```python
from build123d import *

# Parameters (mm, degrees)
BOSS_EXTRU_1_DEPTH      = 40
ESQUISSE2_R             = 8
ENL_V_MAT_EXTRU_1_DEPTH = 190.883457354
ESQUISSE3_R             = 8
ENL_V_MAT_EXTRU_2_DEPTH = 181.562836456
BOSS_EXTRU_2_DEPTH      = 6.35
BOSS_EXTRU_3_START      = 6.35
BOSS_EXTRU_3_DEPTH      = 6.35
ENL_V_START             = -9.5
ENL_V_MAT_EXTRU_3_DEPTH = 9.5
ENL_V_MAT_EXTRU_6_DEPTH = 9.5


with BuildPart() as part:
    # Esquisse1 → Boss.-Extru.1 (new body)
    with BuildSketch(Plane.XY):
        with BuildLine():
            ThreePointArc((-10.389343798, 19.957743747), (6.765880489, 21.458631392), (19.957743747, 10.389343798))
            Line((19.957743747, 10.389343798), (-16.981934979, 81.349806406))
            Line((-16.981934979, 81.349806406), (-28.734828519, 75.231637281))
            Line((-28.734828519, 75.231637281), (-49.975475061, 116.034539653))
            Line((-49.975475061, 116.034539653), (-58.180325268, 111.76336498))
            Line((-58.180325268, 111.76336498), (-10.389343798, 19.957743747))
        make_face()
        with BuildLine():
            ThreePointArc((-22.5, 0), (-19.23551709, 11.672398309), (-10.389343798, 19.957743747))
            Line((-10.389343798, 19.957743747), (-58.180325268, 111.76336498))
            Line((-58.180325268, 111.76336498), (-66.385175475, 107.492190308))
            Line((-66.385175475, 107.492190308), (-45.144528933, 66.689287936))
            Line((-45.144528933, 66.689287936), (-88.25, 44.25))
            Line((-88.25, 44.25), (-88.25, 9.25))
            Line((-88.25, 9.25), (-140, 9.25))
            Line((-140, 9.25), (-140, 0))
            Line((-140, 0), (-22.5, 0))
        make_face()
        with BuildLine():
            Line((-88.25, -22.560492565), (0.015421683, -22.499994715))
            ThreePointArc((0.015421683, -22.499994715), (-15.904449254, -15.915354031), (-22.5, 0))
            Line((-22.5, 0), (-140, 0))
            Line((-140, 0), (-140, -9.25))
            Line((-140, -9.25), (-88.25, -9.25))
            Line((-88.25, -9.25), (-88.25, -22.560492565))
        make_face()
        with BuildLine():
            ThreePointArc((22.5, 0), (21.855196571, 5.347932577), (19.957743747, 10.389343798))
            ThreePointArc((19.957743747, 10.389343798), (6.765880489, 21.458631392), (-10.389343798, 19.957743747))
            Line((-10.389343798, 19.957743747), (-4.386611826, 8.426602915))
            ThreePointArc((-4.386611826, 8.426602915), (4.928345953, 8.121662771), (9.5, 0))
            ThreePointArc((9.5, 0), (0, -9.5), (-9.5, 0))
            Line((-9.5, 0), (-22.5, 0))
            ThreePointArc((-22.5, 0), (-15.904449254, -15.915354031), (0.015421683, -22.499994715))
            ThreePointArc((0.015421683, -22.499994715), (15.915354031, -15.904449254), (22.5, 0))
        make_face()
        with BuildLine():
            Line((-4.386611826, 8.426602915), (-10.389343798, 19.957743747))
            ThreePointArc((-10.389343798, 19.957743747), (-19.23551709, 11.672398309), (-22.5, 0))
            Line((-22.5, 0), (-9.5, 0))
            ThreePointArc((-9.5, 0), (-8.121662771, 4.928345953), (-4.386611826, 8.426602915))
        make_face()
        with BuildLine():
            ThreePointArc((22.5, 0), (21.855196571, 5.347932577), (19.957743747, 10.389343798))
            ThreePointArc((19.957743747, 10.389343798), (6.765880489, 21.458631392), (-10.389343798, 19.957743747))
            Line((-10.389343798, 19.957743747), (-4.386611826, 8.426602915))
            ThreePointArc((-4.386611826, 8.426602915), (4.928345953, 8.121662771), (9.5, 0))
            ThreePointArc((9.5, 0), (0, -9.5), (-9.5, 0))
            Line((-9.5, 0), (-22.5, 0))
            ThreePointArc((-22.5, 0), (-15.904449254, -15.915354031), (0.015421683, -22.499994715))
            ThreePointArc((0.015421683, -22.499994715), (15.915354031, -15.904449254), (22.5, 0))
        make_face()
        with BuildLine():
            Line((-4.386611826, 8.426602915), (-10.389343798, 19.957743747))
            ThreePointArc((-10.389343798, 19.957743747), (-19.23551709, 11.672398309), (-22.5, 0))
            Line((-22.5, 0), (-9.5, 0))
            ThreePointArc((-9.5, 0), (-8.121662771, 4.928345953), (-4.386611826, 8.426602915))
        make_face()
    extrude(amount=BOSS_EXTRU_1_DEPTH)

    # Esquisse2 → Enlèv. mat.-Extru.1 (cut, through all)
    with BuildSketch(Plane(origin=(8.204850207, 4.271174672, 0), x_dir=(0, 0, -1), z_dir=(0.8870108331782228, 0.4617486132350319, 0))):
        with Locations(Location((-20, 106, 0), (0, 0, 90))):
            Circle(ESQUISSE2_R)
        with BuildLine():
            ThreePointArc((-40, 106), (-34.142135624, 120.142135624), (-20, 126))
            Line((-20, 126), (-40, 126))
            Line((-40, 126), (-40, 106))
        make_face()
        with BuildLine():
            ThreePointArc((-20, 126), (-5.857864376, 120.142135624), (0, 106))
            Line((0, 106), (0, 126))
            Line((0, 126), (-20, 126))
        make_face()
    extrude(amount=-ENL_V_MAT_EXTRU_1_DEPTH, mode=Mode.SUBTRACT)

    # Esquisse3 → Enlèv. mat.-Extru.2 (cut, through all)
    with BuildSketch(Plane(origin=(0, 9.25, 0), x_dir=(1, 0, 0), z_dir=(0, 1, 0))):
        with BuildLine():
            ThreePointArc((-140, -20), (-134.142135624, -5.857864376), (-120, 0))
            Line((-120, 0), (-140, 0))
            Line((-140, 0), (-140, -20))
        make_face()
        with BuildLine():
            ThreePointArc((-120, -40), (-134.142135624, -34.142135624), (-140, -20))
            Line((-140, -20), (-140, -40))
            Line((-140, -40), (-120, -40))
        make_face()
        with Locations(Location((-120, -20, 0), (0, 0, 180))):
            Circle(ESQUISSE3_R)
    extrude(amount=-ENL_V_MAT_EXTRU_2_DEPTH, mode=Mode.SUBTRACT)

    # Esquisse4 → Boss.-Extru.2 (add)
    with BuildSketch(Plane.XY.offset(40)):
        with BuildLine():
            ThreePointArc((22.5, 0), (21.855196571, 5.347932577), (19.957743747, 10.389343798))
            ThreePointArc((19.957743747, 10.389343798), (6.765880489, 21.458631392), (-10.389343798, 19.957743747))
            Line((-10.389343798, 19.957743747), (-4.386611826, 8.426602915))
            ThreePointArc((-4.386611826, 8.426602915), (4.928345953, 8.121662771), (9.5, 0))
            ThreePointArc((9.5, 0), (0, -9.5), (-9.5, 0))
            Line((-9.5, 0), (-22.5, 0))
            ThreePointArc((-22.5, 0), (-15.904449254, -15.915354031), (0.015421683, -22.499994715))
            ThreePointArc((0.015421683, -22.499994715), (15.915354031, -15.904449254), (22.5, 0))
        make_face()
        with BuildLine():
            ThreePointArc((22.5, 0), (21.855196571, 5.347932577), (19.957743747, 10.389343798))
            ThreePointArc((19.957743747, 10.389343798), (6.765880489, 21.458631392), (-10.389343798, 19.957743747))
            Line((-10.389343798, 19.957743747), (-4.386611826, 8.426602915))
            ThreePointArc((-4.386611826, 8.426602915), (4.928345953, 8.121662771), (9.5, 0))
            ThreePointArc((9.5, 0), (0, -9.5), (-9.5, 0))
            Line((-9.5, 0), (-22.5, 0))
            ThreePointArc((-22.5, 0), (-15.904449254, -15.915354031), (0.015421683, -22.499994715))
            ThreePointArc((0.015421683, -22.499994715), (15.915354031, -15.904449254), (22.5, 0))
        make_face()
        with BuildLine():
            Line((-4.386611826, 8.426602915), (-10.389343798, 19.957743747))
            ThreePointArc((-10.389343798, 19.957743747), (-19.23551709, 11.672398309), (-22.5, 0))
            Line((-22.5, 0), (-9.5, 0))
            ThreePointArc((-9.5, 0), (-8.121662771, 4.928345953), (-4.386611826, 8.426602915))
        make_face()
    extrude(amount=BOSS_EXTRU_2_DEPTH)

    # Esquisse5 → Boss.-Extru.3 (add)
    with BuildSketch(Plane(origin=(0, 0, 0), x_dir=(-1, 0, 0), z_dir=(0, 0, -1)).offset(BOSS_EXTRU_3_START)):
        with BuildLine():
            ThreePointArc((10.389343798, 19.957743747), (-6.765880489, 21.458631392), (-19.957743747, 10.389343798))
            ThreePointArc((-19.957743747, 10.389343798), (-19.239516139, -11.665805533), (-0.015421683, -22.499994715))
            ThreePointArc((-0.015421683, -22.499994715), (15.904449254, -15.915354031), (22.5, 0))
            Line((22.5, 0), (9.5, 0))
            ThreePointArc((9.5, 0), (-8.121662771, -4.928345953), (4.386611826, 8.426602915))
            Line((4.386611826, 8.426602915), (10.389343798, 19.957743747))
        make_face()
        with BuildLine():
            ThreePointArc((22.5, 0), (19.23551709, 11.672398309), (10.389343798, 19.957743747))
            Line((10.389343798, 19.957743747), (4.386611826, 8.426602915))
            ThreePointArc((4.386611826, 8.426602915), (8.121662771, 4.928345953), (9.5, 0))
            Line((9.5, 0), (22.5, 0))
        make_face()
        with BuildLine():
            ThreePointArc((10.389343798, 19.957743747), (-6.765880489, 21.458631392), (-19.957743747, 10.389343798))
            ThreePointArc((-19.957743747, 10.389343798), (-19.239516139, -11.665805533), (-0.015421683, -22.499994715))
            ThreePointArc((-0.015421683, -22.499994715), (15.904449254, -15.915354031), (22.5, 0))
            Line((22.5, 0), (9.5, 0))
            ThreePointArc((9.5, 0), (-8.121662771, -4.928345953), (4.386611826, 8.426602915))
            Line((4.386611826, 8.426602915), (10.389343798, 19.957743747))
        make_face()
    extrude(amount=-BOSS_EXTRU_3_DEPTH)

    # Esquisse6 → Enlèv. mat.-Extru.3 (cut)
    with BuildSketch(Plane.XY.offset(40).offset(ENL_V_START)):
        with BuildLine():
            Line((19.957743747, 10.389343798), (-12.595323154, 72.923203491))
            Line((-12.595323154, 72.923203491), (-17.695635444, 70.268148965))
            ThreePointArc((-17.695635444, 70.268148965), (-21.385397976, 65.870861212), (-20.885102094, 60.152453117))
            Line((-20.885102094, 60.152453117), (-3.287380782, 26.347545001))
            ThreePointArc((-3.287380782, 26.347545001), (-0.879642567, 23.627512536), (2.52390035, 22.3579947))
            ThreePointArc((2.52390035, 22.3579947), (12.734529101, 18.549441193), (19.957743747, 10.389343798))
        make_face()
        with BuildLine():
            Line((-78.75, -22.553981187), (0.015421683, -22.499994715))
            ThreePointArc((0.015421683, -22.499994715), (-10.566597122, -19.864466398), (-18.666376021, -12.5625))
            ThreePointArc((-18.666376021, -12.5625), (-21.364033316, -10.129718662), (-24.888501361, -9.25))
            Line((-24.888501361, -9.25), (-71.25, -9.25))
            ThreePointArc((-71.25, -9.25), (-76.553300859, -11.446699141), (-78.75, -16.75))
            Line((-78.75, -16.75), (-78.75, -22.553981187))
        make_face()
        with BuildLine():
            Line((-20.950564458, 20.213114599), (-37.294802508, 51.610103772))
            ThreePointArc((-37.294802508, 51.610103772), (-41.69209026, 55.299866303), (-47.410498356, 54.799570422))
            Line((-47.410498356, 54.799570422), (-74.713114599, 40.586728011))
            ThreePointArc((-74.713114599, 40.586728011), (-77.66183903, 37.824946199), (-78.75, 33.934146763))
            Line((-78.75, 33.934146763), (-78.75, 16.75))
            ThreePointArc((-78.75, 16.75), (-76.553300859, 11.446699141), (-71.25, 9.25))
            Line((-71.25, 9.25), (-27.603145707, 9.25))
            ThreePointArc((-27.603145707, 9.25), (-21.191306677, 12.859200564), (-20.950564458, 20.213114599))
        make_face()
    extrude(amount=ENL_V_MAT_EXTRU_3_DEPTH, mode=Mode.SUBTRACT)

    # Esquisse9 → Enlèv. mat.-Extru.6 (cut)
    with BuildSketch(Plane(origin=(0, 0, 0), x_dir=(-1, 0, 0), z_dir=(0, 0, -1))):
        with BuildLine():
            ThreePointArc((-19.957743747, 10.389343798), (-12.734529101, 18.549441193), (-2.52390035, 22.3579947))
            ThreePointArc((-2.52390035, 22.3579947), (0.879642567, 23.627512536), (3.287380782, 26.347545001))
            Line((3.287380782, 26.347545001), (20.885102094, 60.152453117))
            ThreePointArc((20.885102094, 60.152453117), (21.385397976, 65.870861212), (17.695635444, 70.268148965))
            Line((17.695635444, 70.268148965), (12.595323154, 72.923203491))
            Line((12.595323154, 72.923203491), (-19.957743747, 10.389343798))
        make_face()
        with BuildLine():
            Line((47.410498356, 54.799570422), (74.713114599, 40.586728011))
            ThreePointArc((74.713114599, 40.586728011), (77.66183903, 37.824946199), (78.75, 33.934146763))
            Line((78.75, 33.934146763), (78.75, 16.75))
            ThreePointArc((78.75, 16.75), (76.553300859, 11.446699141), (71.25, 9.25))
            Line((71.25, 9.25), (27.603145707, 9.25))
            ThreePointArc((27.603145707, 9.25), (21.191306677, 12.859200564), (20.950564458, 20.213114599))
            Line((20.950564458, 20.213114599), (37.294802508, 51.610103772))
            ThreePointArc((37.294802508, 51.610103772), (41.69209026, 55.299866303), (47.410498356, 54.799570422))
        make_face()
        with BuildLine():
            Line((71.25, -9.25), (24.888501361, -9.25))
            ThreePointArc((24.888501361, -9.25), (21.364033316, -10.129718662), (18.666376021, -12.5625))
            ThreePointArc((18.666376021, -12.5625), (10.566597122, -19.864466398), (-0.015421683, -22.499994715))
            Line((-0.015421683, -22.499994715), (78.75, -22.553981187))
            Line((78.75, -22.553981187), (78.75, -16.75))
            ThreePointArc((78.75, -16.75), (76.553300859, -11.446699141), (71.25, -9.25))
        make_face()
    extrude(amount=-ENL_V_MAT_EXTRU_6_DEPTH, mode=Mode.SUBTRACT)


solid = part.part
```
Part model, mm, in its own coordinate system. A direction names the side the tool comes from. Give positions to 0.01 mm unless a question says otherwise; leave off trailing zeros. Order: outer loops, then holes, each group sorted by start corner. A loop starts at its lowest first (then second) coordinate and runs counter-clockwise, first axis right, second up. Notation, with made-up numbers: M 44.25,35.5 L 86.25,35.5 A22 cw 86.25,57.5 Z; hole C 44,15 d7. An arc over 180 degrees is marked long. Use a Markdown table: item, result. Add a question column.
(1) Mould opens along Y. For faces 1 (the face through (-41.614, 55.275, 35.184)), 2 (the face through (-108, 9.25, 20)), 3 (the face through (-49, -16, 30.5)) say: +Y half, -Y half, draft (parallel to the pull), parting line (faces both ways), or undercut.
(2) Probe line 1 along Z through (x, y) = (-120, 2.5); line 2 along Y through (x, z) = (-52, 34); line 3 along Y through (x, z) = (-43, 31.5). List the from-to ranges inside material, lowest first. Write a range as [from, to].
(3) Saw through at D-D, the plane x = -53. Give the number of separate pieces and of enclosed holes in the cut face, and give its area (3 significant figures).
(4) Saw through at C-C, the plane x = -15. Give the cut face in (y, z), and give its area (3 significant figures).
(5) Saw through at B-B, the plane z = 17. Give the cut face in (x, y), and give its area (3 significant figures).
(6) Saw through at A-A, the plane y = 0. Give the cut face in (x, z).
(7) Drop flat-ended pins along their axis: P1, Ø7.5, axis at y = 27.5, z = 3, coming from the +X side; P2, Ø12, axis at x = -23.5, y = -1, coming from the +Z side; P3, Ø6.5, axis at y = -20.5, z = 5.5, coming from the +X side; P4, Ø5, axis at x = -44.5, z = 35.5, coming from the +Y side. Give the stop position or say it passes through.
(8) 3-axis set-ups, long thin cutter, end or side, ignore diameter. For faces 4 (the face through (-0.922, 23.657, 35.184)), 5 (the face through (-50, 28, 30.5)), 6 (the face through (-4, 44, 9.5)): which of +Z, -Z, +X, -X, +Y, -Y reach the whole face in a straight line?
Answer key:
| question | item | result |
|---|---|---|
| 1 | face 1 | undercut |
| 1 | face 2 | +Y half |
| 1 | face 3 | draft |
| 2 | line 1 | [0, 12], [28, 40] |
| 2 | line 2 | [-9.25, 9.25], [52.41, 63.12], [79.86, 108.54] |
| 2 | line 3 | [-9.25, 9.25], [55.59, 102.63] |
| 3 | separate pieces | 2 |
| 3 | enclosed holes | 1 |
| 3 | area | 3,230 mm^2 |
| 4 | outline | M -22.51,9.5 L -16.77,9.5 L -16.77,-6.35 L 16.77,-6.35 L 16.77,0 L 48.85,0 L 48.85,9.5 L 71.67,9.5 L 71.67,0 L 77.54,0 L 77.54,40 L 71.67,40 L 71.67,30.5 L 48.85,30.5 L 48.85,40 L 16.77,40 L 16.77,46.35 L -16.77,46.35 L -16.77,30.5 L -22.51,30.5 Z |
| 4 | area | 3,890 mm^2 |
| 5 | outline | M -139.77,-9.25 L -127.42,-9.25 L -127.42,9.25 L -139.77,9.25 Z; M -112.58,-9.25 L -88.25,-9.25 L -88.25,-22.56 L 0.02,-22.5 A22.5 ccw 19.96,10.39 L -16.98,81.35 L -28.73,75.23 L -37.32,91.72 L -53.73,83.17 L -45.14,66.69 L -88.25,44.25 L -88.25,9.25 L -112.58,9.25 Z; M -66.28,107.29 L -60.57,96.33 L -44.16,104.87 L -49.87,115.83 Z; hole C 0,0 d19 |
| 5 | area | 9,540 mm^2 |
| 6 | outline | M -120,0 L -22.5,0 L -22.5,-6.35 L -9.5,-6.35 L -9.5,46.35 L -22.5,46.35 L -22.5,40 L -120,40 A20 ccw Z; M 9.5,-6.35 L 22.5,-6.35 L 22.5,46.35 L 9.5,46.35 Z; hole C -120,20 d16 |
| 7 | P1 | x = -1.05 |
| 7 | P2 | z = 46.35 |
| 7 | P3 | x = 14.45 |
| 7 | P4 | y = 110.16 |
| 8 | face 4 | +Z, +X, +Y |
| 8 | face 5 | +Z |
| 8 | face 6 | -Z, +X |
